For this review, take the finished solid that the model builds, in its own axes (mm). Face numbers are marked on the shaded views. Give positions to 0.01 mm unless a question says otherwise; leave off trailing zeros. Write each loop counter-clockwise with the first axis right and the second up, starting at its lowest first coordinate (ties: lowest second). Pieces come first, ordered by that corner, then holes. Notation, with made-up numbers: M 80,45 L 129,45 A12 cw 129,58 Z; hole C -7,32 d5. An arc over 180 degrees is marked long. Use one line per item in the form item = value. Start each with the question number.
Q1. Clearance check with flat-ended pins moving along their axes: pin 1 Ø16.5 at (x, y) = (23.1, -16.5) entering from -Z; pin 2 Ø3 at (x, z) = (6, 1.5) entering from -Y; pin 3 Ø3 at (x, z) = (14.5, 4.5) entering from -Y; pin 4 Ø3 at (y, z) = (-14.5, 6) entering from +X. State where each tip first meets the part, or that it passes through.
Q2. Consider section D-D on x = 30. Write out the cut boundary in (y, z).
Q3. For probe 1 along Y at (x, z) = (0, 5.25); probe 2 along X at (y, z) = (-9.5, 2.75); probe 3 along X at (y, z) = (-22, 5), list the stretches that pass through material, from the lowest coordinate up. Write a range as [from, to].
Q4. Consider section C-C on z = 6. Write out the cut boundary in (x, y) (1 decimal), and give its area (3 significant figures).
Q5. Consider section A-A on x = -6. Write out the cut boundary in (y, z).
Q6. Consider section B-B on y = 0. Write out the cut boundary in (x, z).
Q7. Mouldability with a two-part tool opening along X and no side actions: class the marked faces 1, 2, 3 and 4 as released by +X, released by -X, zero draft, split by the parting line, or undercut.
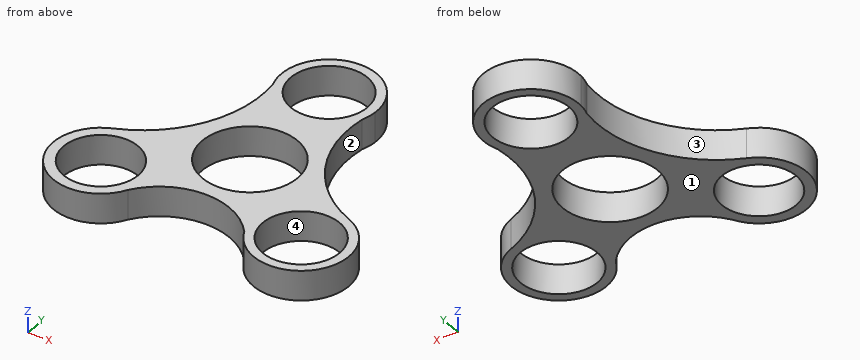
```python
from build123d import *

# Parameters (mm, degrees)
F0_R     = 8.748743
F0_R_2   = 9.032553
F0_R_3   = 11.2
F0_R_4   = 9.0028
F1_DEPTH = 7


with BuildPart() as f1:
    # F0 (on Top) → F1 (new body)
    with BuildSketch(Plane.XY):
        with BuildLine():
            ThreePointArc((11.178943, 26.695394), (10.762369, 25.036023), (10.45059, 23.353811))
            ThreePointArc((10.45059, 23.353811), (10.943067, 24.996637), (11.178943, 26.695394))
        make_face()
        with BuildLine():
            ThreePointArc((-10.576557, 23.697235), (-10.836514, 25.204599), (-11.178943, 26.695394))
            ThreePointArc((-11.178943, 26.695394), (-10.980559, 25.175658), (-10.576557, 23.697235))
        make_face()
        with BuildLine():
            ThreePointArc((27.180357, -6.069851), (13.702991, 5.735114), (10.45059, 23.353811))
            ThreePointArc((10.45059, 23.353811), (10.762369, 25.036023), (11.178943, 26.695394))
            ThreePointArc((11.178943, 26.695394), (0, 38.581858), (-11.178943, 26.695394))
            ThreePointArc((-11.178943, 26.695394), (-10.836514, 25.204599), (-10.576557, 23.697235))
            ThreePointArc((-10.576557, 23.697235), (-13.997206, 5.854713), (-27.703453, -6.069851))
            ThreePointArc((-27.703453, -6.069851), (-31.997535, -23.940002), (-13.746279, -21.778267))
            ThreePointArc((-13.746279, -21.778267), (-0.683408, -14.633163), (12.811986, -20.923272))
            ThreePointArc((12.811986, -20.923272), (31.151847, -24.287939), (27.180357, -6.069851))
        make_face()
        with Locations((-23.624999, -16.500873)):
            Circle(F0_R, mode=Mode.SUBTRACT)
        with Locations((23.101903, -16.500873)):
            Circle(F0_R_2, mode=Mode.SUBTRACT)
        Circle(F0_R_3, mode=Mode.SUBTRACT)
        with Locations((0, 27.381858)):
            Circle(F0_R_4, mode=Mode.SUBTRACT)
    extrude(amount=F1_DEPTH)


solid = f1.part
```
Working result:
q1.pin_1 = through
q1.pin_2 = -16.51
q1.pin_3 = -25.16
q1.pin_4 = 34.29
q2.outline = M -25.32,0 L -22.33,0 L -22.33,7 L -25.32,7 Z; M -10.67,0 L -7.68,0 L -7.68,7 L -10.67,7 Z
q3.probe_1 = [-14.63, -11.2], [11.2, 18.38], [36.38, 38.58]
q3.probe_2 = [-32.37, -28.87], [-18.38, -5.93], [5.93, 17.39], [28.81, 31.84]
q3.probe_3 = [-33.38, -30.43], [-16.82, -13.87], [13.34, 15.94], [30.27, 32.86]
q4.outline = M -27.7,-6.1 A11.2 ccw long -13.7,-21.8 A16.5 cw 12.8,-20.9 A11.2 ccw long 27.2,-6.1 A27.3 cw 10.5,23.4 A11.2 ccw 11.2,26.7 A11.2 ccw long -11.2,26.7 A11.2 ccw -10.6,23.7 A27.8 cw Z; hole C -23.6,-16.5 d17.5; hole C 0,0 d22.4; hole C 0,27.4 d18; hole C 23.1,-16.5 d18.1
q4.area = 1,060 mm²
q5.outline = M -15.7,0 L -9.46,0 L -9.46,7 L -15.7,7 Z; M 9.46,0 L 20.67,0 L 20.67,7 L 9.46,7 Z; M 34.09,0 L 36.84,0 L 36.84,7 L 34.09,7 Z
q6.outline = M -18.5,0 L -11.2,0 L -11.2,7 L -18.5,7 Z; M 11.2,0 L 18.06,0 L 18.06,7 L 11.2,7 Z
q7.face_1 = zero draft
q7.face_2 = released by +X
q7.face_3 = released by -X
q7.face_4 = undercut
